Autodesk Inventor part; units mm, degrees
ref_plane "YZ Plane" through (0, 0, 0) normal (1, 0, 0) x (0, 1, 0)
ref_plane "XZ Plane" through (0, 0, 0) normal (0, 1, 0) x (-1, 0, 0)
ref_plane "XY Plane" through (0, 0, 0) normal (0, 0, 1) x (1, 0, 0)
sketch "草图1" plane through (0, 0, 0) normal (0, 0, 1) x (1, 0, 0)
  line L0 (-195, 100) -> (195, 100)
  line L1 (195, 100) -> (195, -100)
  line L2 (195, -100) -> (-195, -100)
  line L3 (-195, -100) -> (-195, 100)
  line L4 (-273, 0) -> (273, 0)
  line L5 (0, -140) -> (0, 140)
  point P0 (0, 0)
  dimension "d0" = 390
  dimension "d1" = 200
extrude "拉伸1" add sketch "草图1" along normal mid plane 530
sketch "草图2" plane through (195, -100, 265) normal (1, 0, 0) x (0, 0, -1)
  line L0 (0, 200) -> (0, 0)
  line L1 (0, 0) -> (0, 120)
  line L2 (0, 120) -> (480, 0)
  line L3 (530, 0) -> (0, 0)
  line L4 (480, 0) -> (0, 0)
  point P0 (265, 100)
  dimension "d4" = 120
  dimension "d5" = 480
extrude "拉伸2" cut sketch "草图2" against normal through all
shell "抽壳1" thickness 10 removed faces 1 at (-65, 100, 88.3333)
sketch "草图3" plane through (-195, -100, -265) normal (0, -1, 0) x (1, 0, 0)
  line L0 (390, 0) -> (0, 0)
  line L1 (10, 0) -> (380, 0)
  line L2 (380, 0) -> (380, 20)
  line L3 (380, 20) -> (10, 20)
  line L4 (10, 20) -> (10, 0)
  line L5 (195, -106) -> (195, 636)
  line L6 (0, 0) -> (0, 50)
  point P0 (195, 265)
  point P1 (10, 10)
  dimension "d9" = 20
  dimension "d28" = 10
extrude "拉伸3" cut sketch "草图3" against normal through all
sketch "草图4" plane through (195, -100, -265) normal (1, 0, 0) x (0, 0, -1)
  circle A0 centre (-15, 185) radius 7.5
  line L0 (-530, 200) -> (0, 200)
  line L1 (0, 200) -> (0, 0)
  point P0 (-265, 100)
  dimension "d13" = 15
  dimension "d14" = 15
  dimension "d15" = 15
extrude "拉伸4" cut sketch "草图4" against normal through all
sketch "草图6" plane through (185, 27.8078, 255) normal (0, 0, -1) x (-1, 0, 0)
  line L0 (370, 0) -> (0, 0)
  line L1 (370, 72.1922) -> (370, 0)
  line L2 (0, 0) -> (370, 0)
  line L3 (370, 0) -> (370, 75)
  line L4 (370, 75) -> (0, 75)
  line L5 (0, 75) -> (0, 0)
  point P0 (185, -27.8078)
  dimension "d24" = 75
extrude "拉伸6" cut sketch "草图6" against normal through all
sketch "草图10" plane through (-195, -100, -215) normal (0, -0.9701425, 0.2425356) x (1, 0, 0)
  line L0 (0, 494.7727) -> (390, 494.7727)
  line L1 (390, 0) -> (0, 0)
  line L2 (345, 494.7727) -> (325, 494.7727)
  line L3 (325, 494.7727) -> (325, 0)
  line L4 (325, 0) -> (345, 0)
  line L5 (345, 0) -> (345, 494.7727)
  line L6 (390, 494.7727) -> (390, -48.5071)
  point P0 (195, 232.8342)
  point P1 (345, 0)
  dimension "d46" = 20
  dimension "d47" = 45
sketch "草图11" plane through (0, 0, 265) normal (0, 0, 1) x (1, 0, 0)
  line L0 (-195, 20) -> (195, 20)
  line L1 (150, 20) -> (150, 10)
  line L2 (150, -100) -> (150, 20)
  point P0 (0, 0)
  dimension "d50" = 10
sweep "扫掠1" add profiles "草图10" path "草图11" path curves L1 contours L0 L5 L1 L3
sketch "草图14" plane through (130, -100, -215) normal (-1, 0, 0) x (0, 0.2425356, 0.9701425)
  line L0 (-48.5071, 12.1268) -> (0, 0)
  line L1 (0, 0) -> (-2.4254, -9.7014)
  line L2 (-2.4254, -9.7014) -> (36.3803, -19.4029)
  line L3 (36.3803, -19.4029) -> (38.8057, -9.7014)
  line L4 (0, 0) -> (494.7727, 0)
  line L5 (38.8057, -9.7014) -> (0, 0)
  line L6 (0, 0) -> (-2.4254, -9.7014)
  point P0 (232.8342, 44.8691)
  dimension "d54" = 40
extrude "拉伸11" add sketch "草图14" against normal blind 20
sketch "草图15" plane through (0, 0, -265) normal (0, 0, -1) x (-1, 0, 0)
  line L0 (-195, 100) -> (-195, -100)
  line L1 (-185, -100) -> (-185, 100)
  line L2 (-195, 100) -> (-185, 100)
  line L3 (-185, 100) -> (-185, 30)
  line L4 (-185, 30) -> (-195, 30)
  line L5 (-195, 30) -> (-195, 100)
  point P0 (0, 0)
  point P1 (-195, 30)
  dimension "d57" = 70
extrude "拉伸12" add sketch "草图15" along normal blind 40
mirror "镜像3" about plane through (0, 0, 0) normal (1, 0, 0) of "扫掠1", "拉伸11"
mirror "镜像4" about plane through (0, 0, 0) normal (1, 0, 0) of "拉伸12"
sketch "草图5" plane through (-185, -100, -265) normal (1, 0, 0) x (0, 0, -1)
  line L0 (0, 185) -> (15, 185)
  line L1 (15, 185) -> (15, 145)
  line L2 (15, 145) -> (0, 145)
  line L3 (0, 145) -> (0, 185)
  circle A0 centre (-15, 185) radius 7.5
  point P0 (-265, 100)
  dimension "d18" = 15
  dimension "d19" = 40
  dimension "d21" = 0
  dimension "d60" = 15
extrude "拉伸5" cut sketch "草图5" against normal through all contours L0 L1 L2 L3
properties part number "猫砂盆"
CAD build for the part. Positions are in the model's coordinates, mm. A direction names the side the tool comes from. Round coordinates to 2 decimals unless told otherwise and drop trailing zeros. Loops run counter-clockwise (first coordinate to the right, second up) from the corner with the lowest first, then second, coordinate; pieces in that order, holes last. Notation, with made-up numbers: (57, 74) - (111, 74) arc R18 ccw to (111, 88) - close; hole circle Ø10 at (75, 44.25). An arc over 180 degrees is marked (long way). Return JSON: item names as keys, results as strings. Group by question number.
Q1. Band-saw the part on B-B on x = 80. Give the cut face in (y, z).
Q2. Flat gauge pins, fed straight in: pin 1 Ø3 at (x, z) = (-192.5, -270) entering from -Y; pin 2 Ø10 at (x, z) = (51, -27) entering from +Y; pin 3 Ø5 at (x, y) = (143.5, -104) entering from +Z. Where does each tip first touch, or does it go through?
Q3. Band-saw the part on C-C on z = -121. Give the cut face in (x, y).
Q4. Band-saw the part on A-A on y = 36. Give the cut face in (x, z), plus the area to 3 significant figures.
Q5. Tool access for faces 1 (the face through (130, -45, 29)), 2 (the face through (3, -90, -231)), 3 (the face through (172.82, -39.16, 28.36)), 4 (the face through (-172.18, -39.16, 28.36)), 5 (the face through (195, 24, -16)): list every direction of +Z, -Z, +X, -X, +Y, -Y with a clear straight run to the whole face (end or side of a thin tool).
Q6. Drill centre lines: line 1 along X through (y, z) = (13.5, 126); line 2 along Y through (x, z) = (-189, -250); line 3 along Y through (x, z) = (-43, -240). Where is each one in solid material? Low to high. Write a range as [from, to].
Q7. Band-saw the part on D-D on x = -136. Give the cut face in (y, z).
Q8. Two-plate mould, pull along Z, no slides. Class faces 6 (the face through (1.82, -39.16, 28.36)), 7 (the face through (-189.93, 82.13, -256.93)), 8 (the face through (-150, -45, 29)): +Z half, -Z half, draft (parallel to the pull), parting line (faces both ways), or undercut.
Solutions:
{
 "1": {"outline": "(-100, -245) - (-90, -245) - (-90, -216.23) - (27.81, 255) - (27.81, 265) - (20, 265) - (-100, -215) - close"},
 "2": {"pin 1": "stops at y = 30", "pin 2": "stops at y = -41.44", "pin 3": "stops at z = -175"},
 "3": {"outline": "(-195, -76.5) - (-150, -76.5) - (-150, -86.5) - (-130, -86.5) - (-130, -76.5) - (130, -76.5) - (130, -86.5) - (150, -86.5) - (150, -76.5) - (195, -76.5) - (195, 100) - (185, 100) - (185, -66.19) - (-185, -66.19) - (-185, 100) - (-195, 100) - close"},
 "4": {"outline": "(-195, -305) - (-185, -305) - (-185, 265) - (-195, 265) - close; (185, -305) - (195, -305) - (195, 265) - (185, 265) - close", "area": "11,400 mm^2"},
 "5": {"face 1": "+Z, -Y", "face 2": "-Z, +Y", "face 3": "+Z, +X, -Y", "face 4": "+Z, -X, -Y", "face 5": "+Z, -Z, +X, +Y, -Y"},
 "6": {"line 1": "x = [-195, -185], [185, 195]", "line 2": "y = [-100, 77.5], [92.5, 100]", "line 3": "y = [-100, -90]"},
 "7": {"outline": "(-110, -215) - (-100, -215) - (-100, -245) - (-90, -245) - (-90, -216.23) - (27.81, 255) - (27.81, 265) - (10, 265) - (-100, -175) - (-110, -175) - close"},
 "8": {"face 6": "+Z half", "face 7": "undercut", "face 8": "draft"}
}
